Geometry check sheet. Reference: the model listing, model coordinates, mm. A direction names the side the tool comes from. Give positions to 0.01 mm unless a question says otherwise; leave off trailing zeros. Order: outer loops, then holes, each group sorted by start corner. A loop starts at its lowest first (then second) coordinate and runs counter-clockwise, first axis right, second up. Notation, with made-up numbers: M 53.5,79 L 104.5,79 A4 cw 104.5,86 Z; hole C -17,30 d9. An arc over 180 degrees is marked long. Use CSV: the item, a comma, the result in double quotes. Start each with the question number.
from build123d import *

# Parameters (mm, degrees)
SKETCH3_W           = 30
SKETCH3_H           = 12.5
BOSS_EXTRUDE1_DEPTH = 10
SKETCH6_R           = 3.75
SKETCH6_W           = 6.25
SKETCH6_H           = 9
CUT_EXTRUDE2_DEPTH  = 10
SKETCH8_W           = 17.5
SKETCH8_H           = 9
CUT_EXTRUDE4_DEPTH  = 5


with BuildPart() as part:
    # Sketch3 → Boss-Extrude1 (new body)
    with BuildSketch(Plane(origin=(0, 0, 0), x_dir=(1, 0, 0), z_dir=(0, 1, 0))):
        Rectangle(SKETCH3_W, SKETCH3_H)
    extrude(amount=BOSS_EXTRUDE1_DEPTH)

    # Sketch6 → Cut-Extrude2 (cut)
    with BuildSketch(Plane(origin=(0, 10, 0), x_dir=(1, 0, 0), z_dir=(0, 1, 0))):
        with Locations(Location((-4, 1.5, 0), (0, 0, 270))):
            Circle(SKETCH6_R)
        with Locations(Location((4, 1.5, 0), (0, 0, 270))):
            Circle(SKETCH6_R)
        with Locations((-11.875, 1.75)):
            Rectangle(SKETCH6_W, SKETCH6_H)
        with Locations((11.875, 1.75)):
            Rectangle(SKETCH6_W, SKETCH6_H)
    extrude(amount=-CUT_EXTRUDE2_DEPTH, mode=Mode.SUBTRACT)

    # Sketch8 → Cut-Extrude4 (cut)
    with BuildSketch(Plane.XZ):
        with Locations((0, -1.75)):
            Rectangle(SKETCH8_W, SKETCH8_H)
    extrude(amount=-CUT_EXTRUDE4_DEPTH, mode=Mode.SUBTRACT)


solid = part.part
(1) Sectioned sample at C-C on x = -4. Record the cut outline in (y, z), then the cut area to 3 significant figures.
(2) Sectioned sample at D-D on y = 1.5. Record the cut outline in (x, z), then the cut area to 3 significant figures.
(3) Thickness scan on line 1 (X direction, y = 8, z = -1.5); line 2 (X direction, y = 9.25, z = -2.75); line 3 (Z direction, x = 2.75, y = 3.25). Record the ranges inside material, lowest first.
(4) Sectioned sample at A-A on x = 1.75. Record the cut outline in (y, z).
(5) Draft check along X on faces 1 (the face through (0.34, 7.54, -2.31)), 2 (the face through (0, 10, 1)), 3 (the face through (-15, 5, 5)). Enter one of: +X half, -X half, draft (parallel to the pull), parting line (faces both ways), or undercut.
(6) Sectioned sample at B-B on z = -4.5. Record the cut outline in (x, y), then the cut area to 3 significant figures.
(7) Access from +Z, -Z, +X, -X, +Y, -Y to the whole of each face (thin tool, end or side, straight path). Record for faces 4 (the face through (8.75, 8, -2)), 5 (the face through (0, 5, -2)), 6 (the face through (0, 0, 4)), 7 (the face through (-8.75, 8, -2)), 8 (the face through (-0.84, 7.54, 0.52)).
(8) Go/stop test with flat-tipped pins: P1, Ø6, axis at x = -4, z = -1.5, coming from the -Y side; P2, Ø3, axis at y = 7, z = 1, coming from the -X side; P3, Ø1.5, axis at x = -1, z = -4, coming from the -Y side; P4, Ø4, axis at y = 8.5, z = -2.5, coming from the +X side. Record where each tip stops, or that it passes through.
Responses:
1,outline,"M 0,2.75 L 5,2.75 L 5,2.25 L 10,2.25 L 10,6.25 L 0,6.25 Z; M 5,-6.25 L 10,-6.25 L 10,-5.25 L 5,-5.25 Z"
1,area,"42.5 mm2"
2,outline,"M -15,2.75 L 15,2.75 L 15,6.25 L -15,6.25 Z"
2,area,"105 mm2"
3,line 1,"-8.75 to -7.75, -0.25 to 0.25, 7.75 to 8.75"
3,line 2,"-8.75 to -7.54, -0.46 to 0.46, 7.54 to 8.75"
3,line 3,"2.75 to 6.25"
4,outline,"M 0,2.75 L 5,2.75 L 5,1.5 L 10,1.5 L 10,6.25 L 0,6.25 Z; M 5,-6.25 L 10,-6.25 L 10,-4.5 L 5,-4.5 Z"
5,face 1,"undercut"
5,face 2,"draft"
5,face 3,"-X half"
6,outline,"M -8.75,5 L -6.25,5 L -6.25,10 L -8.75,10 Z; M -1.75,5 L 1.75,5 L 1.75,10 L -1.75,10 Z; M 6.25,5 L 8.75,5 L 8.75,10 L 6.25,10 Z"
6,area,"42.5 mm2"
7,face 4,"-Z, +X, +Y, -Y"
7,face 5,"-Z, +X, -X, -Y"
7,face 6,"+Z, -Z, +X, -X, -Y"
7,face 7,"-Z, -X, +Y, -Y"
7,face 8,"+Y, -Y"
8,P1,"through"
8,P2,"x = -8.75"
8,P3,"y = 5"
8,P4,"x = 8.75"
